The listing builds one solid part. Answer for the finished solid, in the listing's coordinates (mm). Round coordinates to 2 decimals unless told otherwise and drop trailing zeros. Write each loop counter-clockwise with the first axis right and the second up, starting at its lowest first coordinate (ties: lowest second). Pieces come first, ordered by that corner, then holes. Notation, with made-up numbers: (66, -1) - (89, -1) arc R13 ccw to (89, 5) - close; hole circle Ø5 at (20, 45). An arc over 180 degrees is marked (long way). Use a Markdown table: item, result. Add a question column.
1) Each of these flat-tipped pins is pushed along its axis until it touches: P1, Ø1.5, axis at y = -37.5, z = 3, coming from the -X side; P2, Ø3, axis at x = 8.125, y = 0, coming from the +Z side. Where does it stop, or does it pass through?
2) A cutting plane is placed at A-A (x = 0). Give the vertices of the cut face in (y, z), then the cut area to 3 significant figures.
3) A cutting plane is placed at D-D (x = 39). Give the vertices of the cut face in (y, z), then the cut area to 3 significant figures.
4) Determine the mould class of faces 1 (the cylindrical face through (-0.867, -3.905, 1.774)), 2 (the flat face through (10, 1, 3.5)), 3 (the cylindrical face through (-10.3, -46.37, 1.73)) for opening direction X: +X half, -X half, draft (parallel to the pull), parting line (faces both ways), or undercut.
5) A cutting plane is placed at C-C (z = 1.1). Give the vertices of the cut face in (x, y) (3 decimals).
6) Find the intervals of material crossed by probe 1 along Y at (x, z) = (0, 1.45); probe 2 along X at (y, z) = (2.5, 2.95); probe 3 along X at (y, z) = (8, 2.6), in increasing order. Write a range as from..to.
```python
from build123d import *

# Parameters (mm, degrees)
F0_R     = 47.5
F1_DEPTH = 3.5
F2_R     = 4
F3_DEPTH = 3.5
F4_R     = 1.625
F5_DEPTH = 3.5


with BuildPart() as f1:
    # F0 (on Top) → F1 (new body)
    with BuildSketch(Plane.XY):
        Circle(F0_R)
    extrude(amount=F1_DEPTH)

    # F2 (on face) → F3 (cut)
    with BuildSketch(Plane.XY.offset(3.5)):
        Circle(F2_R)
    extrude(amount=-F3_DEPTH, mode=Mode.SUBTRACT)

    # F4 (on face) → F5 (cut)
    with BuildSketch(Plane.XY.offset(3.5)):
        with Locations((0, 8.125)):
            Circle(F4_R)
        with Locations((-8.125, 0)):
            Circle(F4_R)
        with Locations((0, -8.125)):
            Circle(F4_R)
        with Locations((8.125, 0)):
            Circle(F4_R)
    extrude(amount=-F5_DEPTH, mode=Mode.SUBTRACT)


solid = f1.part
```
Entries:
| question | item | result |
|---|---|---|
| 1 | P1 | stops at x = -30.09 |
| 1 | P2 | passes through |
| 2 | outline | (-47.5, 0) - (-9.75, 0) - (-9.75, 3.5) - (-47.5, 3.5) - close; (-6.5, 0) - (-4, 0) - (-4, 3.5) - (-6.5, 3.5) - close; (4, 0) - (6.5, 0) - (6.5, 3.5) - (4, 3.5) - close; (9.75, 0) - (47.5, 0) - (47.5, 3.5) - (9.75, 3.5) - close |
| 2 | area | 282 mm² |
| 3 | outline | (-27.12, 0) - (27.12, 0) - (27.12, 3.5) - (-27.12, 3.5) - close |
| 3 | area | 190 mm² |
| 4 | face 1 | undercut |
| 4 | face 2 | draft |
| 4 | face 3 | parting line |
| 5 | outline | circle Ø95 at (0, 0); hole circle Ø3.25 at (-8.125, 0); hole circle Ø8 at (0, 0); hole circle Ø3.25 at (0, -8.125); hole circle Ø3.25 at (0, 8.125); hole circle Ø3.25 at (8.125, 0) |
| 6 | probe 1 | y = -47.5..-9.75, -6.5..-4, 4..6.5, 9.75..47.5 |
| 6 | probe 2 | x = -47.43..-3.12, 3.12..47.43 |
| 6 | probe 3 | x = -46.82..-1.62, 1.62..46.82 |
